from build123d import *

# Parameters (mm, degrees)
CUT_EXTRUDE1_DEPTH      = 111.145358504
CUT_EXTRUDE1_DEPTH_BACK = 111.145358504
SKETCH2_R               = 6


with BuildPart() as part:
    # Sketch1 → Revolve1 (revolve)
    with BuildSketch(Plane(origin=(0, 0, 0), x_dir=(1, 0, 0), z_dir=(0, 1, 0))):
        Polygon((24, 78), (24, 72), (34, 72), (34, 42), (30, 42), (30, 0), (40, 4), (40, 32), (72, 32), (72, 42), (40, 42), (40, 72), (34, 78), align=None)
    revolve(axis=Axis((0, 0, 0), (0, 0, -1)))

    # Sketch2 → Cut-Extrude1 (cut, two sides: drawn at the far end of the back side and taken through both)
    with BuildSketch(Plane(origin=(0, 0, -42), x_dir=(-1, 0, 0), z_dir=(0, 0, -1)).offset(-CUT_EXTRUDE1_DEPTH_BACK)):
        with Locations((0, 58)):
            Circle(SKETCH2_R)
        with Locations((58, 0)):
            Circle(SKETCH2_R)
        with Locations((0, -58)):
            Circle(SKETCH2_R)
        with Locations((-58, 0)):
            Circle(SKETCH2_R)
    extrude(amount=CUT_EXTRUDE1_DEPTH + CUT_EXTRUDE1_DEPTH_BACK, mode=Mode.SUBTRACT)


solid = part.part
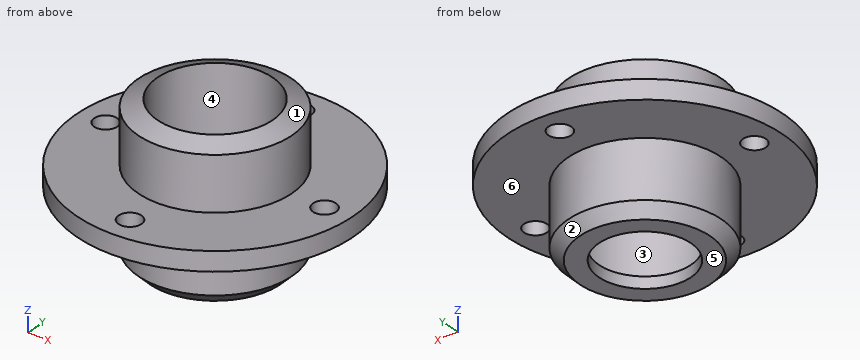
Read the model definition and answer for the solid it produces. Units are mm, in the model's axes. Face numbers are marked on the shaded views. A direction names the side the tool comes from. Give positions to 0.01 mm unless a question says otherwise; leave off trailing zeros. Write each loop counter-clockwise with the first axis right and the second up, starting at its lowest first coordinate (ties: lowest second). Pieces come first, ordered by that corner, then holes. Notation, with made-up numbers: (15, 3) - (46, 3) arc R22 ccw to (46, 25) - close; hole circle Ø10 at (76, 0.5). An arc over 180 degrees is marked (long way). Use CSV: the item, a comma, the result in double quotes. Start each with the question number.
Item 1: Consider line 1 (X direction, y = 0, z = -36); line 2 (Y direction, x = 0, z = -58.5); line 3 (Y direction, x = 0, z = -21). Determine where each line is inside the solid, lowest interval first.
Item 2: Flat-ended cylindrical pins translate along their axes: P1, Ø20.5, axis at x = 13.5, y = 3, coming from the +Z side; P2, Ø6, axis at x = -34, y = -22.5, coming from the +Z side; P3, Ø5, axis at x = 22.5, y = 42.5, coming from the -Z side. Find the tip coordinate at first contact, or state that the pin passes through.
Item 3: The mould has two halves that part along Z. Classify the marked faces 1, 2 and 3: pulls with the +Z half, pulls with the -Z half, needs draft (parallel to the pull), parting line crosses it, or undercut.
Item 4: The part is cut by section A-A, the plane y = 0. Count the separate pieces of the cut face and the enclosed holes in it, and give its area (3 significant figures).
Item 5: The part is cut by section B-B, the plane x = 58. Give the vertices of the cut face in (y, z), and give its area (3 significant figures).
Item 6: The part is cut by section D-D, the plane z = -10.5. Give the vertices of the cut face in (x, y).
Item 7: For the marked faces 4, 5 and 6, determine the directions among +Z, -Z, +X, -X, +Y, -Y from which every point of the face is accessible in a straight line to the end or side of a thin tool.
Taken from the geometry:
1,line 1,"-72 to -64, -52 to -30, 30 to 52, 64 to 72"
1,line 2,"-40 to -34, 34 to 40"
1,line 3,"-40 to -30, 30 to 40"
2,P1,"z = -72"
2,P2,"z = -3.11"
2,P3,"z = -42"
3,face 1,"pulls with the +Z half"
3,face 2,"pulls with the -Z half"
3,face 3,"undercut"
4,separate pieces,"4"
4,enclosed holes,"0"
4,area,"1,720 mm2"
5,outline,"(-42.66, -42) - (-6, -42) - (-6, -32) - (-42.66, -32) - close; (6, -42) - (42.66, -42) - (42.66, -32) - (6, -32) - close"
5,area,"733 mm2"
6,outline,"circle Ø80 at (0, 0); hole circle Ø60 at (0, 0)"
7,face 4,"+Z"
7,face 5,"-Z, +X, -X, +Y, -Y"
7,face 6,"-Z"
